The listing builds one solid part. Answer for the finished solid, in the listing's coordinates (mm). A direction names the side the tool comes from. Round coordinates to 2 decimals unless told otherwise and drop trailing zeros. Write each loop counter-clockwise with the first axis right and the second up, starting at its lowest first coordinate (ties: lowest second). Pieces come first, ordered by that corner, then holes.
(1) The mould has two halves that part along X. Classify faces 4 (the face through (26.074, -32, 4)), 5 (the face through (34, -27.205, 4)), 6 (the face through (-44.176, -20, 4)), 7 (the face through (0, -6, 8)): +X half, -X half, draft (parallel to the pull), parting line (faces both ways), or undercut.
(2) A cutting plane is placed at D-D, the plane z = 5. Give the vertices of the cut face in (x, y), and give its area (3 significant figures).
(3) A cutting plane is placed at C-C, the plane x = 4. Give the vertices of the cut face in (y, z), and give its area (3 significant figures).
(4) A cutting plane is placed at A-A, the plane y = -29.5. Give the vertices of the cut face in (x, z).
(5) For faces 1 (the face through (36, -4.205, 4)), 2 (the face through (-42, -36.205, 4)), 3 (the face through (-23.926, -3, 4)), determine the directions among +Z, -Z, +X, -X, +Y, -Y from which every point of the face is accessible in a straight line to the end or side of a thin tool.
(6) Each of these flat-tipped pins is pushed along its axis until it touches: pin 1 Ø1.6 at (y, z) = (-3, 4) entering from -X; pin 2 Ø2 at (x, z) = (-3, 12) entering from +Y; pin 3 Ø24 at (x, y) = (1.07, -17.21) entering from +Z; pin 4 Ø2.5 at (x, z) = (45, 3) entering from -Y. Where does it stop, or does it pass through?
(7) Find the intervals of material crossed by probe 1 along X at (y, z) = (-32, 3.25); probe 2 along Y at (x, z) = (39, 7.25); probe 3 along Y at (x, z) = (7.5, 3.25), in increasing order.
(8) A cutting plane is placed at B-B, the plane y = -20. Give the vertices of the cut face in (x, z), and give its area (3 significant figures).
from build123d import *

# Parameters (mm, degrees)
SKETCH2_W           = 70
SKETCH2_H           = 51
SKETCH2_R           = 10.5
BOSS_EXTRUDE1_DEPTH = 15
SKETCH3_W           = 10
SKETCH3_H           = 10
CUT_EXTRUDE1_DEPTH  = 54.949798285
CUT_EXTRUDE2_DEPTH  = 7
SKETCH5_W           = 5.25
SKETCH5_H           = 8
BOSS_EXTRUDE2_DEPTH = 23
SKETCH5_3_W         = 5
SKETCH5_3_H         = 8
BOSS_EXTRUDE3_DEPTH = 32
SKETCH5_5_W         = 5
SKETCH5_5_H         = 8
BOSS_EXTRUDE4_DEPTH = 32
SKETCH5_6_W         = 5.25
SKETCH5_6_H         = 8
BOSS_EXTRUDE5_DEPTH = 23


with BuildPart() as part:
    # Sketch2 → Boss-Extrude1 (new body)
    with BuildSketch(Plane.XY):
        with Locations((1.074313409, -11.705169628)):
            Rectangle(SKETCH2_W, SKETCH2_H)
        with Locations((1.074313409, -17.205169628)):
            Circle(SKETCH2_R, mode=Mode.SUBTRACT)
    extrude(amount=BOSS_EXTRUDE1_DEPTH)

    # Sketch3 → Cut-Extrude1 (cut, through all)
    with BuildSketch(Plane.XY.offset(15)):
        with Locations((31.074313409, -32.205169628)):
            Rectangle(SKETCH3_W, SKETCH3_H)
        with Locations((-28.925686591, -32.205169628)):
            Rectangle(SKETCH3_W, SKETCH3_H)
        with BuildLine():
            Line((26.074313409, -4.205169628), (36.074313409, -4.205169628))
            Line((36.074313409, -4.205169628), (36.074313409, 13.794830372))
            Line((36.074313409, 13.794830372), (10.074313409, 13.794830372))
            ThreePointArc((10.074313409, 13.794830372), (21.388021908, 9.108538871), (26.074313409, -2.205169628))
            Line((26.074313409, -2.205169628), (26.074313409, -4.205169628))
        make_face()
        with BuildLine():
            Line((-33.925686591, 13.794830372), (-33.925686591, -4.205169628))
            Line((-33.925686591, -4.205169628), (-23.925686591, -4.205169628))
            Line((-23.925686591, -4.205169628), (-23.925686591, -2.205169628))
            ThreePointArc((-23.925686591, -2.205169628), (-19.23939509, 9.108538871), (-7.925686591, 13.794830372))
            Line((-7.925686591, 13.794830372), (-33.925686591, 13.794830372))
        make_face()
    extrude(amount=-CUT_EXTRUDE1_DEPTH, mode=Mode.SUBTRACT)

    # Sketch4 → Cut-Extrude2 (cut)
    with BuildSketch(Plane.XY.offset(15)):
        with BuildLine():
            Line((-3.925686591, -37.205169628), (-3.925686591, -26.438262285))
            ThreePointArc((-3.925686591, -26.438262285), (-4.299232906, -8.184360352), (11.574313409, -17.205169628))
            ThreePointArc((11.574313409, -17.205169628), (10.095122685, -22.578715943), (6.074313409, -26.438262285))
            Line((6.074313409, -26.438262285), (6.074313409, -37.205169628))
            Line((6.074313409, -37.205169628), (26.074313409, -37.205169628))
            Line((26.074313409, -37.205169628), (26.074313409, -27.205169628))
            Line((26.074313409, -27.205169628), (36.074313409, -27.205169628))
            Line((36.074313409, -27.205169628), (36.074313409, -4.205169628))
            Line((36.074313409, -4.205169628), (26.074313409, -4.205169628))
            Line((26.074313409, -4.205169628), (26.074313409, -2.205169628))
            ThreePointArc((26.074313409, -2.205169628), (21.388021908, 9.108538871), (10.074313409, 13.794830372))
            Line((10.074313409, 13.794830372), (-7.925686591, 13.794830372))
            ThreePointArc((-7.925686591, 13.794830372), (-19.23939509, 9.108538871), (-23.925686591, -2.205169628))
            Line((-23.925686591, -2.205169628), (-23.925686591, -4.205169628))
            Line((-23.925686591, -4.205169628), (-33.925686591, -4.205169628))
            Line((-33.925686591, -4.205169628), (-33.925686591, -27.205169628))
            Line((-33.925686591, -27.205169628), (-23.925686591, -27.205169628))
            Line((-23.925686591, -27.205169628), (-23.925686591, -37.205169628))
            Line((-23.925686591, -37.205169628), (-3.925686591, -37.205169628))
        make_face()
    extrude(amount=-CUT_EXTRUDE2_DEPTH, mode=Mode.SUBTRACT)

    # Sketch5 → Boss-Extrude2 (add)
    with BuildSketch(Plane(origin=(0, -4.205169628, 0), x_dir=(1, 0, 0), z_dir=(0, 1, 0))):
        with Locations((-36.550686591, -4)):
            Rectangle(SKETCH5_W, SKETCH5_H)
    extrude(amount=-BOSS_EXTRUDE2_DEPTH)

    # Sketch5_3 → Boss-Extrude3 (add)
    with BuildSketch(Plane(origin=(0, -4.205169628, 0), x_dir=(1, 0, 0), z_dir=(0, 1, 0))):
        with Locations((-41.675686591, -4)):
            Rectangle(SKETCH5_3_W, SKETCH5_3_H)
    extrude(amount=-BOSS_EXTRUDE3_DEPTH)



with BuildPart() as body_2:
    # Sketch5_5 → Boss-Extrude4 (new body)
    with BuildSketch(Plane(origin=(0, -4.205169628, 0), x_dir=(1, 0, 0), z_dir=(0, 1, 0))):
        with Locations((43.824313409, -4)):
            Rectangle(SKETCH5_5_W, SKETCH5_5_H)
    extrude(amount=-BOSS_EXTRUDE4_DEPTH)


with BuildPart() as part_1:
    add(part.part)

    add(body_2.part)  # Boss-Extrude5 merges body 2
    # Sketch5_6 → Boss-Extrude5 (add)
    with BuildSketch(Plane(origin=(0, -4.205169628, 0), x_dir=(1, 0, 0), z_dir=(0, 1, 0))):
        with Locations((38.699313409, -4)):
            Rectangle(SKETCH5_6_W, SKETCH5_6_H)
    extrude(amount=-BOSS_EXTRUDE5_DEPTH)


solid = part_1.part
Solutions:
1. face 4: undercut
1. face 5: undercut
1. face 6: -X half
1. face 7: draft
2. outline: (-44.18, -36.21) - (-39.18, -36.21) - (-39.18, -27.21) - (-23.93, -27.21) - (-23.93, -37.21) - (26.07, -37.21) - (26.07, -27.21) - (41.32, -27.21) - (41.32, -36.21) - (46.32, -36.21) - (46.32, -4.21) - (26.07, -4.21) - (26.07, -2.21) arc R16 ccw to (10.07, 13.79) - (-7.93, 13.79) arc R16 ccw to (-23.93, -2.21) - (-23.93, -4.21) - (-44.18, -4.21) - close; hole circle Ø21 at (1.07, -17.21)
2. area: 3,120 mm2
3. outline: (-37.21, 0) - (-27.29, 0) - (-27.29, 15) - (-37.21, 15) - close; (-7.12, 0) - (13.79, 0) - (13.79, 8) - (-7.12, 8) - close
3. area: 316 mm2
4. outline: (-44.18, 0) - (-39.18, 0) - (-39.18, 8) - (-44.18, 8) - close; (-23.93, 0) - (26.07, 0) - (26.07, 8) - (6.07, 8) - (6.07, 15) - (-3.93, 15) - (-3.93, 8) - (-23.93, 8) - close; (41.32, 0) - (46.32, 0) - (46.32, 8) - (41.32, 8) - close
5. face 1: +Z, -Z, +X, +Y
5. face 2: +Z, -Z, -X, -Y
5. face 3: +Z, -Z, -X, +Y
6. pin 1: stops at x = -23.93
6. pin 2: stops at y = -26.44
6. pin 3: stops at z = 15
6. pin 4: stops at y = -36.21
7. probe 1: x = -44.18 to -39.18, -23.93 to 26.07, 41.32 to 46.32
7. probe 2: y = -27.21 to -4.21
7. probe 3: y = -37.21 to -25.51, -8.9 to 13.79
8. outline: (-44.18, 0) - (-9.05, 0) - (-9.05, 8) - (-44.18, 8) - close; (11.2, 0) - (46.32, 0) - (46.32, 8) - (11.2, 8) - close
8. area: 562 mm2
